CAD build for the part. Positions are in the model's coordinates, mm. Face numbers are marked on the shaded views. A direction names the side the tool comes from. Give positions to 0.01 mm unless a question says otherwise; leave off trailing zeros. Order: outer loops, then holes, each group sorted by start corner. A loop starts at its lowest first (then second) coordinate and runs counter-clockwise, first axis right, second up. Notation, with made-up numbers: (-27.75, 19.25) -> (-9.75, 19.25) arc R31 ccw to (-9.75, 52.25) -> close; hole circle Ø3 at (9, 14). An arc over 180 degrees is marked (long way). Use one line per item in the form item = value. Start each with the question number.
1) Drop flat-ended pins along their axis: P1, Ø9, axis at x = -1.5, z = -22, coming from the -Y side; P2, Ø5, axis at x = 1.5, y = 8.5, coming from the +Z side; P3, Ø6, axis at y = 7, z = -11.5, coming from the +X side; P4, Ø3.5, axis at x = 0, y = 2, coming from the +Z side. Give the stop position or say it passes through.
2) Cut at D-D, the plane y = 9.5. Give the cut face in (x, z), and give its area (3 significant figures).
3) Mould opens along Z. For the marked faces 1, 2 and 3 say: pulls with the +Z half, pulls with the -Z half, needs draft (parallel to the pull), parting line crosses it, or undercut.
4) Probe line 1 (X direction, y = 10.9, z = 20); line 2 (X direction, y = 2.25, z = -10); line 3 (Y direction, x = 3.75, z = 4). List the from-to ranges inside material, lowest first.
5) Cut at A-A, the plane y = 12. Give the cut face in (x, z).
6) Cut at B-B, the plane z = 20. Give the cut face in (x, y), and give its area (3 significant figures).
7) Tool access for the marked faces 4, 5, 6 and 7: list every direction of +Z, -Z, +X, -X, +Y, -Y with a clear straight run to the whole face (end or side of a thin tool).
8) Cut at C-C, the plane x = -3.75. Give the cut face in (y, z), and give its area (3 significant figures).
from build123d import *

# Parameters (mm, degrees)
SKETCH_1_W          = 20
SKETCH_1_H          = 10
EXTRUDE_1_DEPTH     = 3
SKETCH_2_W          = 8
SKETCH_2_H          = 3
EXTRUDE_2_DEPTH     = 5
SKETCH_3_R          = 1.75
CUT_EXTRUDE_1_DEPTH = 10
FILLET_1_R          = 5
FILLET_2_R          = 5


with BuildPart() as part:
    # 草图1 → 凸台-拉伸1 (new body)
    with BuildSketch(Plane(origin=(0, 0, 0), x_dir=(1, 0, 0), z_dir=(0, 1, 0))):
        Rectangle(SKETCH_1_W, SKETCH_1_H)
        with BuildLine():
            ThreePointArc((-6.5, -1.75), (-8.25, 0), (-6.5, 1.75))
            Line((-6.5, 1.75), (6.5, 1.75))
            ThreePointArc((6.5, 1.75), (7.737436867, 1.237436867), (8.25, 0))
            ThreePointArc((8.25, 0), (7.737436867, -1.237436867), (6.5, -1.75))
            Line((6.5, -1.75), (-6.5, -1.75))
        make_face(mode=Mode.SUBTRACT)
    extrude(amount=EXTRUDE_1_DEPTH)

    # 草图2 → 凸台-拉伸2 (add, symmetric)
    with BuildSketch(Plane(origin=(0, 0, 0), x_dir=(0, 0, -1), z_dir=(1, 0, 0))):
        with Locations((-21, 11.5)):
            Rectangle(SKETCH_2_W, SKETCH_2_H)
        Polygon((-12, 3), (-5, 3), (-5, 0), (-15, 0), (-17, 10), (-17, 13), (-16, 13), align=None)
        Polygon((16, 13), (17, 13), (17, 10), (15, 0), (5, 0), (5, 3), (12, 3), align=None)
        with Locations((21, 11.5)):
            Rectangle(SKETCH_2_W, SKETCH_2_H)
    extrude(amount=EXTRUDE_2_DEPTH, both=True)

    # 草图3 → 切除-拉伸1 (cut)
    with BuildSketch(Plane(origin=(0, 13, 0), x_dir=(1, 0, 0), z_dir=(0, 1, 0))):
        with Locations(Location((0, 20, 0), (0, 0, 270))):
            Circle(SKETCH_3_R)
        with Locations(Location((0, -20, 0), (0, 0, 270))):
            Circle(SKETCH_3_R)
    extrude(amount=-CUT_EXTRUDE_1_DEPTH, mode=Mode.SUBTRACT)

    # 圆角1
    fillet_1_edges = [part.edges().sort_by_distance(p)[0] for p in [
        (0, 0, 15),
        (0, 3, 12),
        (0, 3, -12),
        (0, 0, -15),
    ]]
    fillet(fillet_1_edges, radius=FILLET_1_R)

    # 圆角2
    fillet_2_edges = [part.edges().sort_by_distance(p)[0] for p in [
        (-10, 1.5, 5),
        (-10, 1.5, -5),
        (10, 1.5, -5),
        (10, 1.5, 5),
    ]]
    fillet(fillet_2_edges, radius=FILLET_2_R - 0.0001)  # a hair under: the kernel refuses the full size


solid = part.part
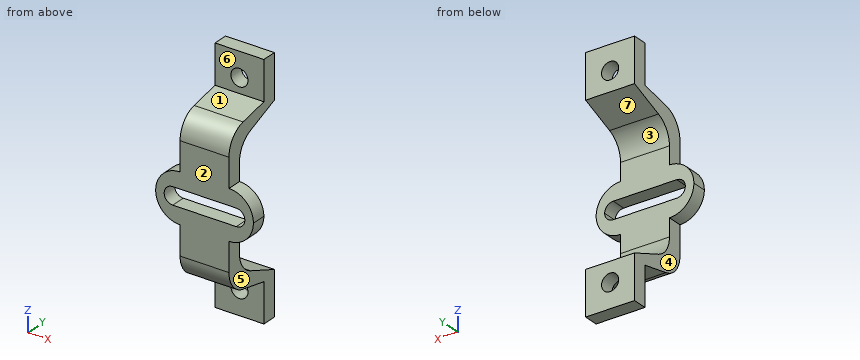
Result:
q1.P1 = 10
q1.P2 = 25
q1.P3 = 5
q1.P4 = 15.74
q2.outline = (-5, -16.9) -> (5, -16.9) -> (5, -14.6) -> (-5, -14.6) -> close; (-5, 14.6) -> (5, 14.6) -> (5, 16.9) -> (-5, 16.9) -> close
q2.area = 46.0 mm²
q3.face_1 = pulls with the +Z half
q3.face_2 = needs draft
q3.face_3 = undercut
q4.line_1 = -5 to -1.75, 1.75 to 5
q4.line_2 = -5 to 5
q4.line_3 = 0 to 3
q5.outline = (-5, -25) -> (5, -25) -> (5, -15.6) -> (-5, -15.6) -> close; (-5, 15.6) -> (5, 15.6) -> (5, 25) -> (-5, 25) -> close; hole circle Ø3.5 at (0, -20); hole circle Ø3.5 at (0, 20)
q6.outline = (-5, 10) -> (-1.75, 10) -> (-1.75, 13) -> (-5, 13) -> close; (1.75, 10) -> (5, 10) -> (5, 13) -> (1.75, 13) -> close
q6.area = 19.5 mm²
q7.face_4 = -Z, -X, +Y, -Y
q7.face_5 = -Z, +X, +Y, -Y
q7.face_6 = +Z, +X, -X, -Y
q7.face_7 = +X, -X, +Y
q8.outline = (0, -10.9) arc R5 ccw to (4.02, -15.8) -> (10, -17) -> (10, -25) -> (13, -25) -> (13, -16) -> (6.14, -13.26) arc R5 cw to (3, -8.61) -> (3, -1.75) -> (0, -1.75) -> close; (0, 1.75) -> (3, 1.75) -> (3, 8.61) arc R5 cw to (6.14, 13.26) -> (13, 16) -> (13, 25) -> (10, 25) -> (10, 17) -> (4.02, 15.8) arc R5 ccw to (0, 10.9) -> close
q8.area = 177 mm²
